Design review of the part built by this model. Coordinates are the model's own, in mm. A direction names the side the tool comes from. Coordinates: 2 decimals unless noted, no trailing zeros.
Q1. The part is to be moulded in two halves that separate along X. For faces 1 (the cylindrical face through (102.493, 9.86, -0.605)), 2 (the flat face through (75, 3, 7.031)), 3 (the flat face through (-1, 0, 25)), 4 (the flat face through (75, 3, -7.031)), say which applies: released by +X, released by -X, zero draft, split by the parting line, or undercut.
Q2. For faces 5 (the flat face through (-82, 13, 5)), 6 (the flat face through (-8, 10, -21.4)), 7 (the flat face through (85.057, 3.204, 5.194)), list the 3-axis set-ups (+Z, -Z, +X, -X, +Y, -Y) from which the entire face can be reached by the end or side of a thin tool; tool diameter is ignored.
Q3. Take a section at A-A, the plane y = 11. State how many separate pieces and enclosed holes the cut face has, plus the area to 3 significant figures.
Q4. For pin 1 Ø1 at (y, z) = (15.5, -14) entering from +X; pin 2 Ø5.5 at (x, z) = (88, 0) entering from -Y; pin 3 Ø11 at (x, z) = (62, 0) entering from -Y; pin 4 Ø11 at (x, z) = (-85, -4.5) entering from +Y, all flat-tipped, find the tip position at first contact; note any pin that passes through.
Q5. For L1, parallel to Z at x = 75, y = 15.75; L2, parallel to X at y = 17, z = -13; L3, parallel to X at y = 17, z = -3, list the stretches that pass through material, from the lowest coordinate up.
from build123d import *

# Parameters (mm, degrees)
SKETCH1_W             = 150
SKETCH1_H             = 55
BOSS_EXTRUDE1_DEPTH   = 20
SKETCH2_W             = 27.5
SKETCH2_H             = 55
BOSS_EXTRUDE2_DEPTH   = 20
M8_CLEARANCE_HOLE1_D  = 10
M6_CLEARANCE_HOLE1_D  = 7
FILLET1_R             = 10
SKETCH11_W            = 42.4
SKETCH11_H            = 42.4
CUT_EXTRUDE1_DEPTH    = 108.993055332
SKETCH12_R            = 4
CUT_EXTRUDE2_DEPTH    = 108.993055332
SKETCH13_W            = 47.6
SKETCH13_H            = 42.8
CUT_EXTRUDE3_DEPTH    = 108.993055332
CUT_EXTRUDE4_DEPTH    = 6.5
SKETCH15_R            = 11.1
CUT_EXTRUDE5_DEPTH    = 7
F_3_0MM_DOWEL_HOLE1_D = 3.2


with BuildPart() as part:
    # Sketch1 → Boss-Extrude1 (new body)
    with BuildSketch(Plane(origin=(0, 0, 0), x_dir=(1, 0, 0), z_dir=(0, 1, 0))):
        Rectangle(SKETCH1_W, SKETCH1_H)
    extrude(amount=BOSS_EXTRUDE1_DEPTH)

    # Sketch2 → Boss-Extrude2 (add)
    with BuildSketch(Plane.XZ):
        with Locations((-88.75, 0)):
            Rectangle(SKETCH2_W, SKETCH2_H)
        with BuildLine():
            Line((75, 27.5), (75, -27.5))
            ThreePointArc((75, -27.5), (102.5, 0), (75, 27.5))
        make_face()
    extrude(amount=-BOSS_EXTRUDE2_DEPTH)

    # M8 Clearance Hole1 (through all)
    with Locations(Plane(origin=(0, 0, 0), x_dir=(-1, 0, 0), z_dir=(0, -1, 0))):
        with Locations((-75, 0)):
            Hole(M8_CLEARANCE_HOLE1_D / 2)

    # M6 Clearance Hole1 (through all)
    with Locations(Plane(origin=(0, 20, 0), x_dir=(1, 0, 0), z_dir=(0, 1, 0))):
        with Locations((75, 13), (62, 0), (88, 0), (75, -13)):
            Hole(M6_CLEARANCE_HOLE1_D / 2)

    # Fillet1
    fillet1_edges = [part.edges().sort_by_distance(p)[0] for p in [
        (-102.5, 10, -27.5),
        (-102.5, 10, 27.5),
    ]]
    fillet(fillet1_edges, radius=FILLET1_R)

    # Sketch11 → Cut-Extrude1 (cut, through all)
    with BuildSketch(Plane.XZ):
        with Locations((-10, 0)):
            Rectangle(SKETCH11_W, SKETCH11_H)
    extrude(amount=-CUT_EXTRUDE1_DEPTH, mode=Mode.SUBTRACT)

    # Sketch12 → Cut-Extrude2 (cut, through all)
    with BuildSketch(Plane(origin=(0, 20, 0), x_dir=(1, 0, 0), z_dir=(0, 1, 0))):
        with Locations(Location((-82.5, 0, 0), (0, 0, 270))):
            Circle(SKETCH12_R)
    extrude(amount=-CUT_EXTRUDE2_DEPTH, mode=Mode.SUBTRACT)

    # Sketch13 → Cut-Extrude3 (cut, through all)
    with BuildSketch(Plane.XZ):
        with Locations((-7.6, 0)):
            Rectangle(SKETCH13_W, SKETCH13_H)
    extrude(amount=-CUT_EXTRUDE3_DEPTH, mode=Mode.SUBTRACT)

    # Sketch14 → Cut-Extrude4 (cut)
    with BuildSketch(Plane.XZ):
        Polygon((93.969119661, 3.446272843), (88, 6.892545686), (82.030880339, 3.446272843), (82.030880339, -3.446272843), (88, -6.892545686), (93.969119661, -3.446272843), align=None)
        Polygon((71.553727157, 18.969119661), (68.107454314, 13), (71.553727157, 7.030880339), (78.446272843, 7.030880339), (81.892545686, 13), (78.446272843, 18.969119661), align=None)
        Polygon((78.446272843, -18.969119661), (81.892545686, -13), (78.446272843, -7.030880339), (71.553727157, -7.030880339), (68.107454314, -13), (71.553727157, -18.969119661), align=None)
        Polygon((56.030880339, -3.446272843), (62, -6.892545686), (67.969119661, -3.446272843), (67.969119661, 3.446272843), (62, 6.892545686), (56.030880339, 3.446272843), align=None)
    extrude(amount=-CUT_EXTRUDE4_DEPTH, mode=Mode.SUBTRACT)

    # Sketch15 → Cut-Extrude5 (cut)
    with BuildSketch(Plane(origin=(0, 20, 0), x_dir=(1, 0, 0), z_dir=(0, 1, 0))):
        with Locations(Location((-82.5, 0, 0), (0, 0, 270))):
            Circle(SKETCH15_R)
    extrude(amount=-CUT_EXTRUDE5_DEPTH, mode=Mode.SUBTRACT)

    # Ø3.0mm Dowel Hole1 (through all)
    with Locations(Plane(origin=(0, 0, 0), x_dir=(-1, 0, 0), z_dir=(0, -1, 0))):
        with Locations((51.4, 0)):
            Hole(F_3_0MM_DOWEL_HOLE1_D / 2)


solid = part.part
Responses:
1. face 1: released by +X
1. face 2: undercut
1. face 3: zero draft
1. face 4: undercut
2. face 5: +Y
2. face 6: +Y, -Y
2. face 7: -Y
3. separate pieces: 1
3. enclosed holes: 8
3. area: 8,580 mm2
4. pin 1: stops at x = 98.96
4. pin 2: passes through
4. pin 3: stops at y = 6.5
4. pin 4: stops at y = 13
5. L1: z = -27.5 to -16.5, -9.5 to -5, 5 to 9.5, 16.5 to 27.5
5. L2: x = -102.5 to -31.4, 16.2 to 71.5, 78.5 to 99.23
5. L3: x = -102.5 to -93.19, -71.81 to -31.4, 16.2 to 60.2, 63.8 to 71, 79 to 86.2, 89.8 to 102.34
